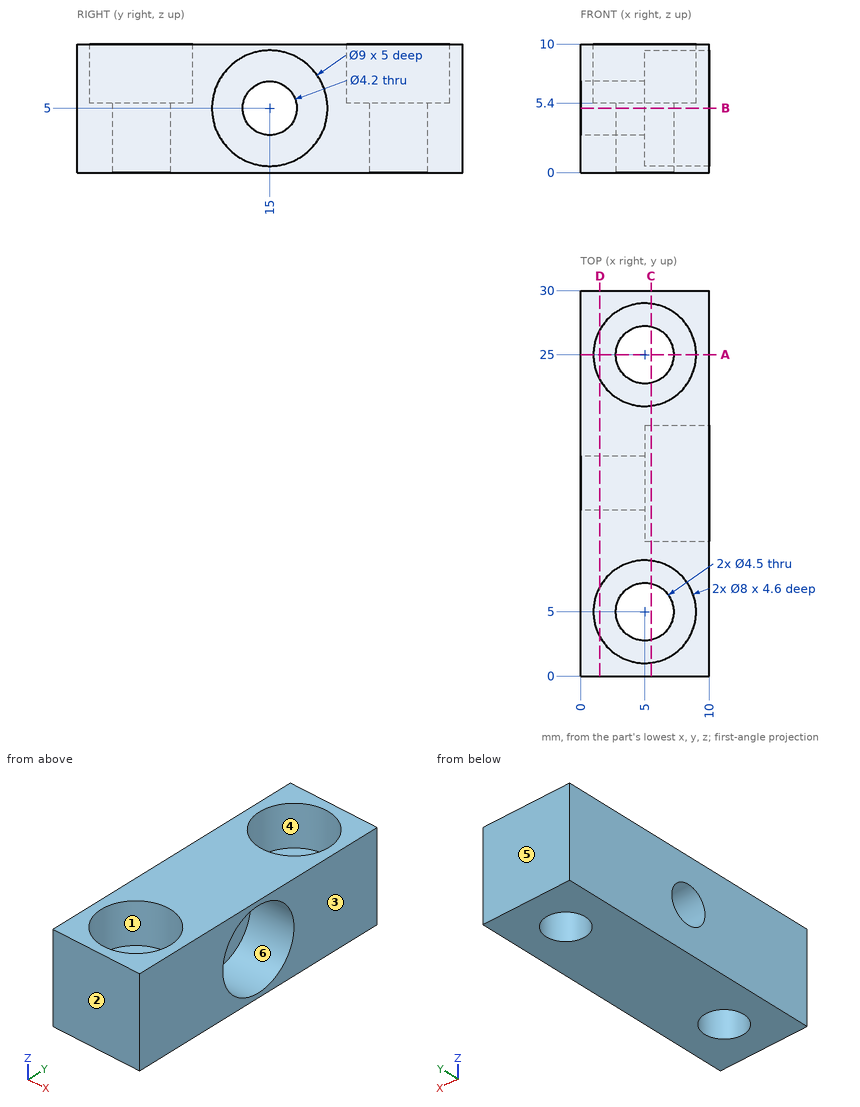
Print and shaded views of the part. All mm, measured from the part's lowest x, y and z. A direction names the side the tool comes from. Coordinates: 2 decimals unless noted, no trailing zeros. Loops run counter-clockwise (first coordinate to the right, second up) from the corner with the lowest first, then second, coordinate; pieces in that order, holes last. Notation, with made-up numbers: M 30,35.25 L 78,35.25 A22 cw 78,68.25 Z; hole C 46.5,61 d3. An arc over 180 degrees is marked long. Use a Markdown table: item, result. Add a question column.
Q1. Which spindle directions (+Z, -Z, +X, -X, +Y, -Y) get a long thin tool onto all of the face, cutting with end or side? Do the marked faces 4, 5 and 6. Say none if no direction does.
Q2. Cut at A-A (y = 25). Write the cut outline in (x, z), and give its area (3 significant figures).
Q3. Cut at C-C (x = 5.5). Write the cut outline in (y, z), and give its area (3 significant figures).
Q4. Mould opens along Y. For the marked faces 1, 2 and 3 say: +Y half, -Y half, draft (parallel to the pull), parting line (faces both ways), or undercut.
Q5. Cut at D-D (x = 1.5). Write the cut outline in (y, z), and give its area (3 significant figures).
Q6. Pin check, flat tips, straight feed: P1, Ø4, axis at x = 6.5, z = 3.5, coming from the -Y side; P2, Ø5, axis at x = 5, y = 25, coming from the +Z side; P3, Ø2.5, axis at y = 16, z = 6.5, coming from the +X side. Stop position of each tip, or through.
Q7. Probe L1, parallel to Z at x = 5.75, y = 15.25; L2, parallel to Y at x = 7.5, z = 8; L3, parallel to Y at x = 8.15, z = 5. List the from-to ranges inside material, lowest first.
Q8. Cut at B-B (z = 5). Write the cut outline in (x, y).
Worked out:
| question | item | result |
|---|---|---|
| 1 | face 4 | +Z |
| 1 | face 5 | +Z, -Z, +X, -X, +Y |
| 1 | face 6 | +X |
| 2 | outline | M 0,0 L 2.75,0 L 2.75,5.4 L 1,5.4 L 1,10 L 0,10 Z; M 7.25,0 L 10,0 L 10,10 L 9,10 L 9,5.4 L 7.25,5.4 Z |
| 2 | area | 38.9 mm2 |
| 3 | outline | M 0,0 L 2.81,0 L 2.81,5.4 L 1.03,5.4 L 1.03,10 L 0,10 Z; M 7.19,0 L 22.81,0 L 22.81,5.4 L 21.03,5.4 L 21.03,10 L 8.97,10 L 8.97,5.4 L 7.19,5.4 Z; M 27.19,0 L 30,0 L 30,10 L 28.97,10 L 28.97,5.4 L 27.19,5.4 Z; hole C 15,5 d9 |
| 3 | area | 116 mm2 |
| 4 | face 1 | undercut |
| 4 | face 2 | -Y half |
| 4 | face 3 | draft |
| 5 | outline | M 0,0 L 30,0 L 30,10 L 26.94,10 L 26.94,5.4 L 23.06,5.4 L 23.06,10 L 6.94,10 L 6.94,5.4 L 3.06,5.4 L 3.06,10 L 0,10 Z; hole C 15,5 d4.2 |
| 5 | area | 251 mm2 |
| 6 | P1 | stops at y = 0 |
| 6 | P2 | stops at z = 5.4 |
| 6 | P3 | stops at x = 5 |
| 7 | L1 | z = 0 to 0.51, 9.49 to 10 |
| 7 | L2 | y = 0 to 1.88, 8.12 to 11.65, 18.35 to 21.88, 28.12 to 30 |
| 7 | L3 | y = 0 to 10.5, 19.5 to 30 |
| 8 | outline | M 0,0 L 10,0 L 10,10.5 L 5,10.5 L 5,12.9 L 0,12.9 Z; M 0,17.1 L 5,17.1 L 5,19.5 L 10,19.5 L 10,30 L 0,30 Z; hole C 5,5 d4.5; hole C 5,25 d4.5 |
